from build123d import *

# Parameters (mm, degrees)
BOSS_EXTRU_1_DEPTH      = 20
ESQUISSE2_R             = 20
BOSS_EXTRU_2_DEPTH      = 50
ESQUISSE3_R             = 12.5
ENL_V_MAT_EXTRU_1_DEPTH = 83.487366196


with BuildPart() as part:
    # Esquisse1 → Boss.-Extru.1 (new, symmetric)
    with BuildSketch(Plane.XY):
        with BuildLine():
            Line((-17.5, 49.896071292), (-34.700811909, 19.896071292))
            ThreePointArc((-34.700811909, 19.896071292), (0, -40), (34.700811909, 19.896071292))
            Line((34.700811909, 19.896071292), (17.5, 49.896071292))
            ThreePointArc((17.5, 49.896071292), (0, 60.034703013), (-17.5, 49.896071292))
        make_face()
    extrude(amount=BOSS_EXTRU_1_DEPTH, both=True)

    # Esquisse2 → Boss.-Extru.2 (add)
    with BuildSketch(Plane(origin=(0, 0, 0), x_dir=(1, 0, 0), z_dir=(0, 1, 0))):
        with Locations(Location((0, 0, 0), (0, 0, 270))):
            Circle(ESQUISSE2_R)
    extrude(amount=-BOSS_EXTRU_2_DEPTH)

    # Esquisse3 → Enlèv. mat.-Extru.1 (cut, through all)
    with BuildSketch(Plane.XY.offset(20)):
        Circle(ESQUISSE3_R)
    extrude(amount=-ENL_V_MAT_EXTRU_1_DEPTH, mode=Mode.SUBTRACT)

    # Esquisse5 → Enlèvement de matière-Révolution1 (revolve, cut)
    with BuildSketch(Plane.XY, mode=Mode.PRIVATE) as enl_vement_de_mati_re_r_volution1_sk:
        Polygon((0, -50), (0, -20), (10, -25.773502692), (10, -50), align=None)
    revolve(enl_vement_de_mati_re_r_volution1_sk.sketch.rotate(Axis((0, -50, 0), (0, 1, 0)), 90), axis=Axis((0, -50, 0), (0, 1, 0)), mode=Mode.SUBTRACT)


solid = part.part
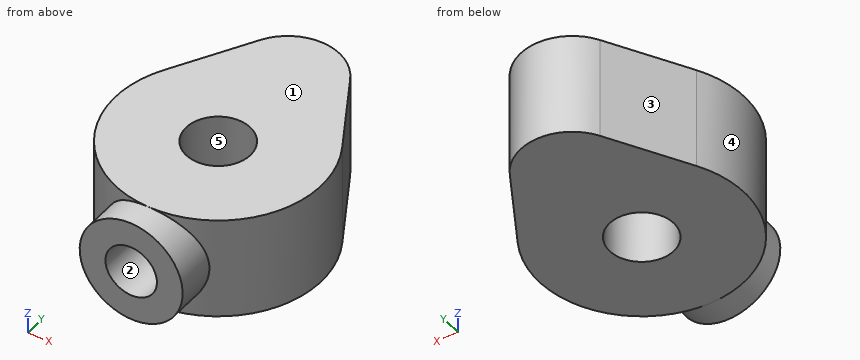
Geometry check sheet. Reference: the model listing, model coordinates, mm. Face numbers are marked on the shaded views. A direction names the side the tool comes from. Round coordinates to 2 decimals unless told otherwise and drop trailing zeros. Order: outer loops, then holes, each group sorted by start corner. A loop starts at its lowest first (then second) coordinate and runs counter-clockwise, first axis right, second up. Notation, with made-up numbers: M 60,-14 L 96,-14 A9 cw 96,-2 Z; hole C 29.25,11.5 d8. An arc over 180 degrees is marked long. Answer in a Markdown table with one row per item.
(1) Sectioned sample at B-B, the plane y = -38. Record the cut outline in (x, z), and give its area (3 significant figures).
Responses:
| item | result |
|---|---|
| outline | M -12.49,-20 L 12.49,-20 L 12.49,-15.62 A20 ccw 12.49,15.62 L 12.49,20 L -12.49,20 L -12.49,15.62 A20 ccw -12.49,-15.62 Z; hole C 0,0 d20 |
| area | 1,010 mm² |
(2) Tool access check on the marked faces 1 and 2. Record the directions out of +Z, -Z, +X, -X, +Y, -Y that give a thin tool (end or side, any length) a straight path to the whole face; none if there is none.
Responses:
| item | result |
|---|---|
| face 1 | +Z, +X, -X, +Y, -Y |
| face 2 | -Y |
(3) Sectioned sample at D-D, the plane y = 43. Record the cut outline in (x, z).
Responses:
| item | result |
|---|---|
| outline | M -21.45,-20 L 21.45,-20 L 21.45,20 L -21.45,20 Z |
(4) Scan lines: probe 1 along X at (y, z) = (0, -0.5); probe 2 along Z at (x, y) = (-0.5, -26.5); probe 3 along Y at (x, z) = (0, 8). Record each from-to range of solid material in increasing order. Write a range as from..to.
Responses:
| item | result |
|---|---|
| probe 1 | x = -40..-12.5, 12.5..40 |
| probe 2 | z = -20..-9.99, 9.99..20 |
| probe 3 | y = -24.62..-12.5, 12.5..60.03 |
(5) Go/stop test with flat-tipped pins: P1, Ø2, axis at x = 29.5, z = -5.5, coming from the -Y side; P2, Ø2, axis at y = -27, z = 2, coming from the +X side; P3, Ø1, axis at x = -28.5, z = 5, coming from the +Y side; P4, Ø5, axis at x = -7.5, y = -7, coming from the -Z side. Record where each tip stops, or that it passes through.
Responses:
| item | result |
|---|---|
| P1 | stops at y = -28.07 |
| P2 | stops at x = 30.4 |
| P3 | stops at y = 31.58 |
| P4 | stops at z = -20 |
(6) Sectioned sample at C-C, the plane x = 26. Record the cut outline in (y, z).
Responses:
| item | result |
|---|---|
| outline | M -30.4,-20 L 35.07,-20 L 35.07,20 L -30.4,20 Z |
(7) Sectioned sample at A-A, the plane y = 0. Record the cut outline in (x, z).
Responses:
| item | result |
|---|---|
| outline | M -40,-20 L -12.5,-20 L -12.5,20 L -40,20 Z; M 12.5,-20 L 40,-20 L 40,20 L 12.5,20 Z |
(8) Draft check along Y on the marked faces 3, 4 and 5. Enter one of: released by +Y, released by -Y, zero draft, split by the parting line, or undercut.
Responses:
| item | result |
|---|---|
| face 3 | released by +Y |
| face 4 | split by the parting line |
| face 5 | undercut |
